Read the model definition and answer for the solid it produces. Units are mm, in the model's axes. Face numbers are marked on the shaded views. A direction names the side the tool comes from. Give positions to 0.01 mm unless a question says otherwise; leave off trailing zeros. Write each loop counter-clockwise with the first axis right and the second up, starting at its lowest first coordinate (ties: lowest second). Pieces come first, ordered by that corner, then holes. Notation, with made-up numbers: M 50,27 L 92,27 A26 ccw 92,54 Z; hole C 78.25,-24.5 d5. An arc over 180 degrees is marked long. Use a Markdown table: item, result. Add a question column.
Item 1: A cutting plane is placed at A-A on x = 0. Determine the outline of the cut face in (y, z).
Item 2: Given P1, Ø1.5, axis at y = -1, z = -4.5, coming from the -X side; P2, Ø0.6, axis at x = 0, z = 1.5, coming from the -Y side; P3, Ø1.5, axis at x = -1, z = 0.5, coming from the +Y side, each flat-ended and moving along its own axis, determine where each tip first touches the part or whether it passes through.
Item 3: Consider probe 1 along Z at (x, y) = (-0.1, -1.95); probe 2 along Z at (x, y) = (1.75, 0.2); probe 3 along X at (y, z) = (0.7, -5.75). Determine where each line is inside the solid, lowest interval first. Write a range as [from, to].
Item 4: A cutting plane is placed at B-B on y = 0. Determine the outline of the cut face in (x, z), then the cut area to 3 significant figures.
Item 5: For the marked faces 5 and 6, determine the directions among +Z, -Z, +X, -X, +Y, -Y from which every point of the face is accessible in a straight line to the end or side of a thin tool.
Item 6: The mould has two halves that part along Y. Classify the marked faces 1, 2, 3 and 4: pulls with the +Y half, pulls with the -Y half, needs draft (parallel to the pull), parting line crosses it, or undercut.
Item 7: A cutting plane is placed at C-C on z = -0.25. Determine the outline of the cut face in (x, y).
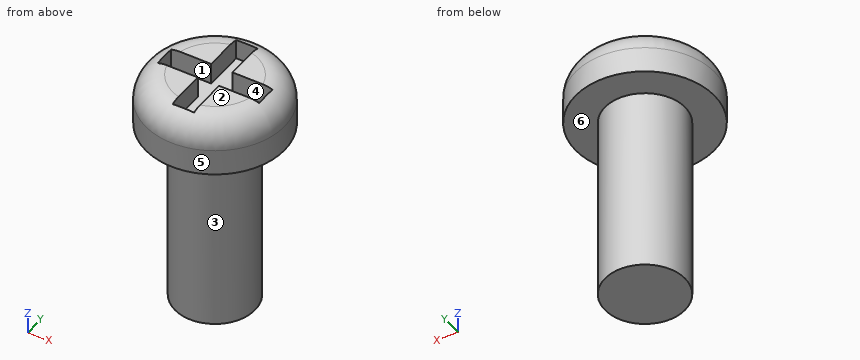
from build123d import *

# Parameters (mm, degrees)
SKETCH1_R           = 2.6
BOSS_EXTRUDE1_DEPTH = 1.97
SKETCH2_R           = 1.5
BOSS_EXTRUDE2_DEPTH = 7
FILLET1_R           = 1
CUT_EXTRUDE1_DEPTH  = 0.8


with BuildPart() as part:
    # Sketch1 → Boss-Extrude1 (new body)
    with BuildSketch(Plane.XY):
        Circle(SKETCH1_R)
    extrude(amount=BOSS_EXTRUDE1_DEPTH)

    # Sketch2 → Boss-Extrude2 (add)
    with BuildSketch(Plane(origin=(0, 0, 0), x_dir=(-1, 0, 0), z_dir=(0, 0, -1))):
        Circle(SKETCH2_R)
    extrude(amount=BOSS_EXTRUDE2_DEPTH)

    # Fillet1
    fillet1_edges = [part.edges().sort_by_distance(p)[0] for p in [
        (-2.6, 0, 1.97),
    ]]
    fillet(fillet1_edges, radius=FILLET1_R)

    # Sketch3 → Cut-Extrude1 (cut)
    with BuildSketch(Plane.XY.offset(1.97)):
        Polygon((-0.392282833, 0.394745479), (-0.392282833, 1.894745479), (0.407717167, 1.894745479), (0.407717167, 0.394745479), (1.907717167, 0.394745479), (1.907717167, -0.405254521), (0.407717167, -0.405254521), (0.407717167, -1.905254521), (-0.392282833, -1.905254521), (-0.392282833, -0.405254521), (-1.892282833, -0.405254521), (-1.892282833, 0.394745479), align=None)
    extrude(amount=-CUT_EXTRUDE1_DEPTH, mode=Mode.SUBTRACT)


solid = part.part
Filled in:
| question | item | result |
|---|---|---|
| 1 | outline | M -2.6,0 L -1.5,0 L -1.5,-7 L 1.5,-7 L 1.5,0 L 2.6,0 L 2.6,0.97 A1 ccw 1.89,1.93 L 1.89,1.17 L -1.91,1.17 L -1.91,1.92 A1 ccw -2.6,0.97 Z |
| 2 | P1 | x = -1.48 |
| 2 | P2 | y = -2.57 |
| 2 | P3 | y = 2.59 |
| 3 | probe 1 | [0, 1.91] |
| 3 | probe 2 | [0, 1.17] |
| 3 | probe 3 | [-1.33, 1.33] |
| 4 | outline | M -2.6,0 L -1.5,0 L -1.5,-7 L 1.5,-7 L 1.5,0 L 2.6,0 L 2.6,0.97 A1 ccw 1.91,1.92 L 1.91,1.17 L -1.89,1.17 L -1.89,1.93 A1 ccw -2.6,0.97 Z |
| 4 | area | 27.8 mm² |
| 5 | face 5 | +Z, -Z |
| 5 | face 6 | -Z |
| 6 | face 1 | undercut |
| 6 | face 2 | needs draft |
| 6 | face 3 | parting line crosses it |
| 6 | face 4 | undercut |
| 7 | outline | C 0,0 d3 |
